Check sheet for the modelled part. Datum: model origin and axes. Units: mm. Face numbers are marked on the shaded views. A direction names the side the tool comes from. Round coordinates to 2 decimals unless told otherwise and drop trailing zeros. Order: outer loops, then holes, each group sorted by start corner. A loop starts at its lowest first (then second) coordinate and runs counter-clockwise, first axis right, second up. Notation, with made-up numbers: M -30.5,22 L -7.5,22 A17 cw -7.5,50 Z; hole C -10,63 d11. An arc over 180 degrees is marked long. One line per item, written item: value. Start each with the question number.
(1) Cross-section at A-A, the plane z = 6. Enter the section's corners in (x, y), and give its area (3 significant figures).
(2) Cross-section at D-D, the plane y = -2. Enter the section's corners in (x, z), and give its area (3 significant figures).
(3) Depth check by flat-ended pin: pin 1 Ø9.5 at (y, z) = (-11.5, 29.5) entering from +X; pin 2 Ø11 at (x, y) = (-31, -10.5) entering from +Z; pin 3 Ø4 at (x, y) = (32.766, -9.525) entering from -Z; pin 4 Ø5.5 at (y, z) = (-10, 15) entering from -X. Enter the tip coordinate at first touch or a pass-through.
(4) Release check for a two-part mould opening along X. For the marked faces 1, 2, 3 and 4 record: released by +X, released by -X, zero draft, split by the parting line, or undercut.
(5) Thickness scan on L1, parallel to X at y = -4.5, z = 17.5; L2, parallel to X at y = -16.75, z = 3; L3, parallel to Z at x = -5.5, y = -10.25. Record the ranges inside material, lowest first.
(6) Cross-section at C-C, the plane y = -8.5. Enter the section's corners in (x, z) (3 decimals), and give its area (3 significant figures).
(7) Cross-section at B-B, the plane x = 33.5. Enter the section's corners in (y, z) (3 decimals), and give its area (3 significant figures).
(8) Access from +Z, -Z, +X, -X, +Y, -Y to the whole of each face (thin tool, end or side, straight path). Record for the marked faces 5, 6 and 7.
from build123d import *

# Parameters (mm, degrees)
F1_W     = 20.701
F1_H     = 3.81
F1_W_2   = 3.81
F1_H_2   = 32.639
F1_W_3   = 16.51
F2_DEPTH = 19.05
F3_R     = 2.54
F4_DEPTH = 3.811
F5_R     = 5.08
F6_DEPTH = 1.905


with BuildPart() as f2:
    # F1 (on Front) → F2 (new body)
    with BuildSketch(Plane.XZ):
        with Locations((10.3505, 38.354)):
            Rectangle(F1_W, F1_H)
        with Locations((22.606, 38.354)):
            Rectangle(F1_W_2, F1_H)
        with Locations((22.606, 20.1295)):
            Rectangle(F1_W_2, F1_H_2)
        with Locations((22.606, 1.905)):
            Rectangle(F1_W_2, F1_H)
        with Locations((32.766, 1.905)):
            Rectangle(F1_W_3, F1_H)
    extrude(amount=F2_DEPTH)

    # F3 (on face) → F4 (cut, through all)
    with BuildSketch(Plane.XY.offset(3.81)):
        with Locations((32.766, -9.525)):
            Circle(F3_R)
    extrude(amount=-F4_DEPTH, mode=Mode.SUBTRACT)

    # F5 (on face) → F6 (cut)
    with BuildSketch(Plane.XY.offset(3.81)):
        with Locations((32.766, -9.525)):
            Circle(F5_R)
    extrude(amount=-F6_DEPTH, mode=Mode.SUBTRACT)

    # F7: F2 across plane


with BuildPart() as f2_1:
    add(f2.part)
    add(f2.part.mirror(Plane.YZ))


solid = f2_1.part
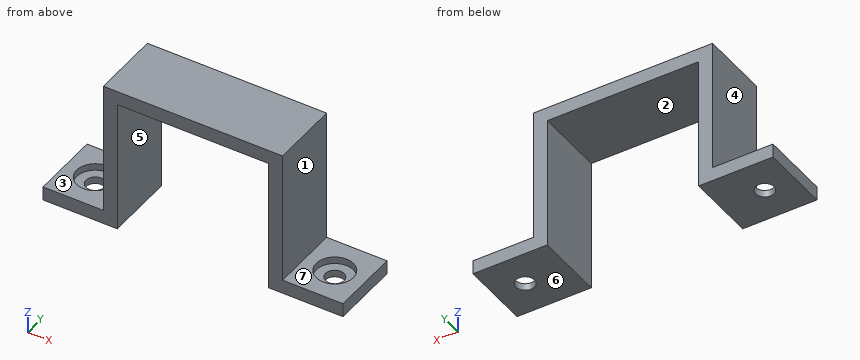
Values found:
1. outline: M -24.51,-19.05 L -20.7,-19.05 L -20.7,0 L -24.51,0 Z; M 20.7,-19.05 L 24.51,-19.05 L 24.51,0 L 20.7,0 Z
1. area: 145 mm^2
2. outline: M -41.02,0 L -20.7,0 L -20.7,36.45 L 20.7,36.45 L 20.7,0 L 41.02,0 L 41.02,3.81 L 24.51,3.81 L 24.51,40.26 L -24.51,40.26 L -24.51,3.81 L -41.02,3.81 Z
2. area: 590 mm^2
3. pin 1: x = 24.51
3. pin 2: z = 3.81
3. pin 3: through
3. pin 4: x = -24.51
4. face 1: released by +X
4. face 2: undercut
4. face 3: zero draft
4. face 4: released by -X
5. L1: -24.51 to -20.7, 20.7 to 24.51
5. L2: -41.02 to -20.7, 20.7 to 41.02
5. L3: 36.45 to 40.26
6. outline: M -41.021,0 L -35.09,0 L -35.09,1.905 L -37.742,1.905 L -37.742,3.81 L -41.021,3.81 Z; M -30.442,0 L -20.701,0 L -20.701,36.449 L 20.701,36.449 L 20.701,0 L 30.442,0 L 30.442,1.905 L 27.79,1.905 L 27.79,3.81 L 24.511,3.81 L 24.511,40.259 L -24.511,40.259 L -24.511,3.81 L -27.79,3.81 L -27.79,1.905 L -30.442,1.905 Z; M 35.09,0 L 41.021,0 L 41.021,3.81 L 37.742,3.81 L 37.742,1.905 L 35.09,1.905 Z
6. area: 535 mm^2
7. outline: M -19.05,0 L -11.957,0 L -11.957,1.905 L -14.552,1.905 L -14.552,3.81 L -19.05,3.81 Z; M -7.093,0 L 0,0 L 0,3.81 L -4.498,3.81 L -4.498,1.905 L -7.093,1.905 Z
7. area: 44.2 mm^2
8. face 5: -Z, +Y, -Y
8. face 6: -Z, +X, -X, +Y, -Y
8. face 7: +Z, +X, +Y, -Y
